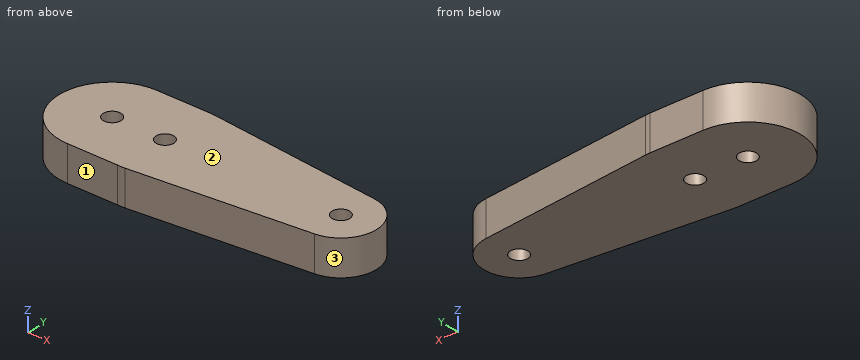
from build123d import *

# Parameters (mm, degrees)
SKETCH1_R           = 2.5
BOSS_EXTRUDE1_DEPTH = 5


with BuildPart() as part:
    # Sketch1 → Boss-Extrude1 (new, symmetric)
    with BuildSketch(Plane.XY):
        with BuildLine():
            Line((1.370602209, 14.9582984), (51.004064798, 9.949465005))
            ThreePointArc((51.004064798, 9.949465005), (60, 0), (51.004064798, -9.949465005))
            Line((51.004064798, -9.949465005), (1.370602209, -14.9582984))
            ThreePointArc((1.370602209, -14.9582984), (0.289429434, -15.018171395), (-0.793247409, -15))
            Line((-0.793247409, -15), (-15, -15))
            ThreePointArc((-15, -15), (-29.999996344, -0.010472716), (-15.020945427, 14.999985376))
            Line((-15.020945427, 14.999985376), (0, 15.020960071))
            ThreePointArc((0, 15.020960071), (0.686016928, 15.005286476), (1.370602209, 14.9582984))
        make_face()
        with Locations((-15, 0)):
            Circle(SKETCH1_R, mode=Mode.SUBTRACT)
        Circle(SKETCH1_R, mode=Mode.SUBTRACT)
        with Locations((50, 0)):
            Circle(SKETCH1_R, mode=Mode.SUBTRACT)
    extrude(amount=BOSS_EXTRUDE1_DEPTH, both=True)


solid = part.part
Verification items for the finished model (mm, model axes). Face numbers are marked on the shaded views. Coordinates: 2 decimals unless noted, no trailing zeros. Order: outer loops, then holes, each group sorted by start corner. A loop starts at its lowest first (then second) coordinate and runs counter-clockwise, first axis right, second up. Notation, with made-up numbers: M -17,58 L 19,58 A22 cw 19,76 Z; hole C 35,35 d5. An arc over 180 degrees is marked long. One line per item, written item: value. Start each with the question number.
Item 1: Gauge pin test, flat ends, axial feed: pin 1 (1 mm diameter, centred on x = 2.5, z = -2.5, fed in from +Y); pin 2 (1.5 mm diameter, centred on x = -13, z = 0, fed in from +Y); pin 3 (1.5 mm diameter, centred on y = 4.5, z = 0.5, fed in from +X). Record the tip position at first contact, or that the pin passes through.
Item 2: Sectioned sample at D-D (x = 35). Enter the section's corners in (y, z), then the cut area to 3 significant figures.
Item 3: Scan lines: probe 1 along Y at (x, z) = (0, -0.25); probe 2 along X at (y, z) = (2, 3.75); probe 3 along X at (y, z) = (-0.5, 1). Record each from-to range of solid material in increasing order.
Item 4: Sectioned sample at B-B (z = -0.5). Enter the section's corners in (x, y), then the cut area to 3 significant figures.
Item 5: Sectioned sample at A-A (y = 0). Enter the section's corners in (x, z).
Item 6: Sectioned sample at C-C (x = 50). Enter the section's corners in (y, z), then the cut area to 3 significant figures.
Item 7: Mould release check, pull along Y, two halves, no side actions. Record for the marked faces 1, 2 and 3: released by +Y, released by -Y, zero draft, split by the parting line, or undercut.
Conclusion:
1. pin 1: stops at y = 14.89
1. pin 2: stops at y = 15
1. pin 3: stops at x = 59.27
2. outline: M -11.56,-5 L 11.56,-5 L 11.56,5 L -11.56,5 Z
2. area: 231 mm^2
3. probe 1: y = -15.02 to -2.5, 2.5 to 15.02
3. probe 2: x = -29.87 to -16.5, -13.5 to -1.5, 1.5 to 48.5, 51.5 to 59.8
3. probe 3: x = -29.99 to -17.45, -12.55 to -2.45, 2.45 to 47.55, 52.45 to 59.99
4. outline: M -15.02,15 A15 ccw -15,-15 L -0.79,-15 A15.02 ccw 1.37,-14.96 L 51,-9.95 A10 ccw 51,9.95 L 1.37,14.96 A15.02 ccw 0,15.02 Z; hole C -15,0 d5; hole C 0,0 d5; hole C 50,0 d5
4. area: 2,160 mm^2
5. outline: M -30,-5 L -17.5,-5 L -17.5,5 L -30,5 Z; M -12.5,-5 L -2.5,-5 L -2.5,5 L -12.5,5 Z; M 2.5,-5 L 47.5,-5 L 47.5,5 L 2.5,5 Z; M 52.5,-5 L 60,-5 L 60,5 L 52.5,5 Z
6. outline: M -10.05,-5 L -2.5,-5 L -2.5,5 L -10.05,5 Z; M 2.5,-5 L 10.05,-5 L 10.05,5 L 2.5,5 Z
6. area: 151 mm^2
7. face 1: released by -Y
7. face 2: zero draft
7. face 3: split by the parting line
